Verification items for this drawing (mm, ordinates from the low corner). A direction names the side the tool comes from. Give positions to 0.01 mm unless a question says otherwise; leave off trailing zeros. Write each loop counter-clockwise with the first axis right and the second up, starting at its lowest first coordinate (ties: lowest second). Pieces come first, ordered by that corner, then holes. Notation, with made-up numbers: (24, 14) -> (81, 14) arc R11 ccw to (81, 24) -> close; hole circle Ø5 at (7.25, 37.5). An arc over 180 degrees is marked (long way). One line per item, written item: value.
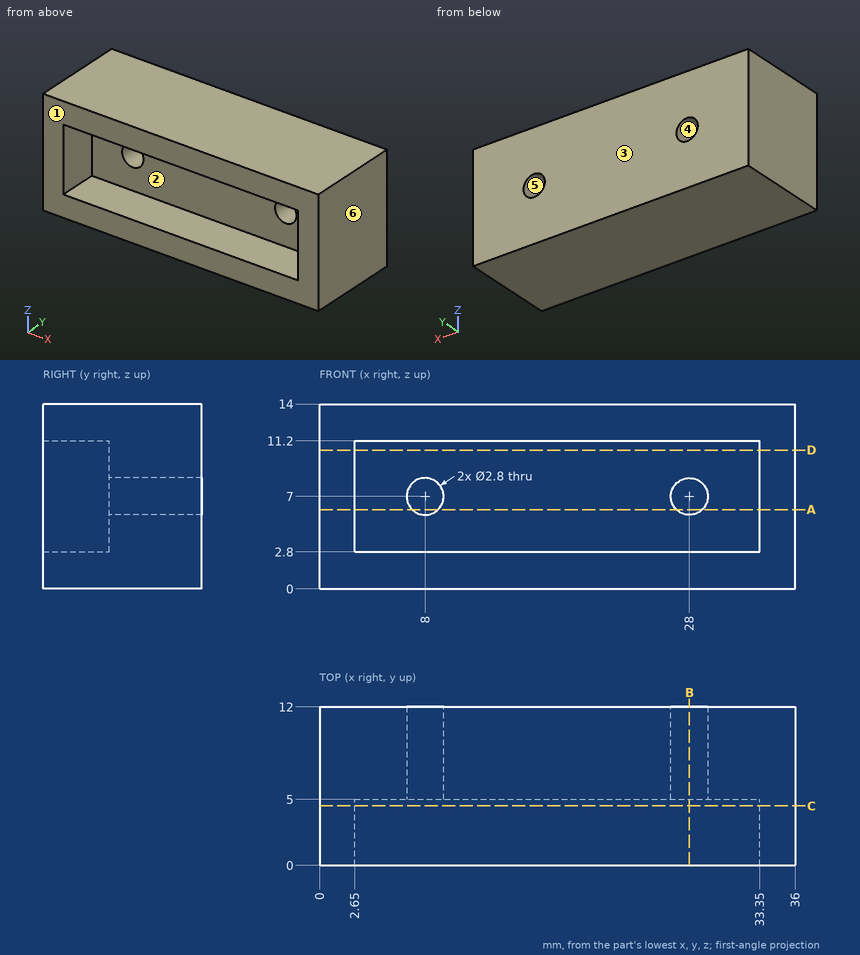
1) Depth check by flat-ended pin: pin 1 Ø3 at (x, z) = (28, 7) entering from +Y; pin 2 Ø4 at (x, z) = (23, 5) entering from -Y. Enter the tip coordinate at first touch or a pass-through.
Verdict:
pin 1: y = 12
pin 2: y = 5
2) Scan lines: probe 1 along X at (y, z) = (1, 7.5); probe 2 along Z at (x, y) = (28, 6.5); probe 3 along Z at (x, y) = (23, 3.25). Record each from-to range of solid material in increasing order.
Verdict:
probe 1: 0 to 2.65, 33.35 to 36
probe 2: 0 to 5.6, 8.4 to 14
probe 3: 0 to 2.8, 11.2 to 14
3) Sectioned sample at C-C on y = 4.5. Record the cut outline in (x, z), plus the area to 3 significant figures.
Verdict:
outline: (0, 0) -> (36, 0) -> (36, 14) -> (0, 14) -> close; hole (2.65, 2.8) -> (33.35, 2.8) -> (33.35, 11.2) -> (2.65, 11.2) -> close
area: 246 mm^2
4) Sectioned sample at D-D on z = 10.5. Record the cut outline in (x, y), plus the area to 4 significant figures.
Verdict:
outline: (0, 0) -> (2.65, 0) -> (2.65, 5) -> (33.35, 5) -> (33.35, 0) -> (36, 0) -> (36, 12) -> (0, 12) -> close
area: 278.5 mm^2
5) Tool access check on the marked faces 1 and 2. Record the directions out of +Z, -Z, +X, -X, +Y, -Y that give a thin tool (end or side, any length) a straight path to the whole face; none if there is none.
Verdict:
face 1: +Z, -Z, +X, -X, -Y
face 2: -Y
6) Mould release check, pull along X, two halves, no side actions. Record for the marked faces 3, 4, 5 and 6: released by +X, released by -X, zero draft, split by the parting line, or undercut.
Verdict:
face 3: zero draft
face 4: undercut
face 5: undercut
face 6: released by +X
7) Sectioned sample at B-B on x = 28. Record the cut outline in (y, z), plus the area to 3 significant figures.
Verdict:
outline: (0, 0) -> (12, 0) -> (12, 5.6) -> (5, 5.6) -> (5, 2.8) -> (0, 2.8) -> close; (0, 11.2) -> (5, 11.2) -> (5, 8.4) -> (12, 8.4) -> (12, 14) -> (0, 14) -> close
area: 106 mm^2
8) Sectioned sample at A-A on z = 6. Record the cut outline in (x, y).
Verdict:
outline: (0, 0) -> (2.65, 0) -> (2.65, 5) -> (7.02, 5) -> (7.02, 12) -> (0, 12) -> close; (8.98, 5) -> (27.02, 5) -> (27.02, 12) -> (8.98, 12) -> close; (28.98, 5) -> (33.35, 5) -> (33.35, 0) -> (36, 0) -> (36, 12) -> (28.98, 12) -> close
